```python
from build123d import *

# Parameters (mm, degrees)
EXTRUDE001_DEPTH               = 300
EXTRUDE002_DEPTH               = 300
EXTRUDE002_PLACEMENT_ANGLE     = 180
EXTRUDE004_DEPTH               = 2
EXTRUDE003_DEPTH               = 2
SKETCH_W                       = 449.952683
SKETCH_H                       = 299.978927
EXTRUDE_DEPTH                  = 2
FUSION_PLACEMENT_ANGLE         = 180
BASEFEATURE001_PLACEMENT_ANGLE = 180
POCKET001_DEPTH                = 825.012353
EXTRUDE005_DEPTH               = 450
POCKET_DEPTH                   = 250
POCKET002_DEPTH                = 500


with BuildPart() as right:
    # Wire → Extrude001 (new body)
    with BuildSketch(Plane(origin=(218.5150455, 150, 100.0712645), x_dir=(1, 0, 0), z_dir=(0, 1, 0))):
        Polygon((6.4963075, 100.0846805), (-3.4711005, 100.0846805), (-3.4711005, -98.1016935), (-6.4963075, -98.1016935), (-6.4963075, -98.7846775), (-5.4995125, -98.7846775), (-5.4995125, -99.4307345), (-6.4963075, -99.4307345), (-6.4963075, -100.0846805), (6.4963075, -100.0846805), (-1.4816445, -9.9001025), (-1.4816445, 10.1120285), (6.4963075, 98.0725005), align=None)
    extrude(amount=-EXTRUDE001_DEPTH)


with BuildPart() as left:
    # Wire001 → Extrude002 (new body)
    with BuildSketch(Plane(origin=(218.5150455, 150, 100.0712645), x_dir=(1, 0, 0), z_dir=(0, 1, 0))):
        Polygon((6.4963075, 100.0846805), (-3.4711005, 100.0846805), (-3.4711005, -98.1016935), (-6.4963075, -98.1016935), (-6.4963075, -98.7846775), (-5.4995125, -98.7846775), (-5.4995125, -99.4307345), (-6.4963075, -99.4307345), (-6.4963075, -100.0846805), (6.4963075, -100.0846805), (-1.4816445, -9.9001025), (-1.4816445, 10.1120285), (6.4963075, 98.0725005), align=None)
    extrude(amount=-EXTRUDE002_DEPTH)


with BuildPart() as left_1:
    # Extrude002 placement: moved
    add(left.part.rotate(Axis((0, 0, 0), (0, 0, 1)), EXTRUDE002_PLACEMENT_ANGLE))


with BuildPart() as inner_back_holder:
    # Sketch002 → Extrude004 (new body)
    with BuildSketch(Plane.XZ.offset(150)):
        Polygon((-213.019012, 3.99983), (-213.019012, 192.972672), (-216.785446, 192.972672), (-216.785446, 0.188954), (216.195801, 0.188954), (216.195801, 193.007004), (213.035522, 193.006973), (213.035522, 3.99983), align=None)
    extrude(amount=-EXTRUDE004_DEPTH)


with BuildPart() as inner_back_holder_1:
    # Extrude004 placement: moved
    add(inner_back_holder.part.moved(Location((0, 3, 0))))


with BuildPart() as outer_back_holder:
    # Sketch001 → Extrude003 (new body)
    with BuildSketch(Plane.XZ.offset(150)):
        Polygon((-213.019012, 3.99983), (-213.019012, 192.972672), (-216.785446, 192.972672), (-216.785446, 0.188954), (216.195801, 0.188954), (216.195801, 193.007004), (213.035522, 193.006973), (213.035522, 3.99983), align=None)
    extrude(amount=-EXTRUDE003_DEPTH)


with BuildPart() as main_body:
    # Sketch → Extrude (new body)
    with BuildSketch(Plane.XY):
        with Locations((-0.0037765, 0.0109025)):
            Rectangle(SKETCH_W, SKETCH_H)
    extrude(amount=EXTRUDE_DEPTH)

    # Fusion: union Right, Left, Inner-Back-Holder, Outer-Back-Holder
    add(right.part)
    add(left_1.part)
    add(inner_back_holder_1.part)
    add(outer_back_holder.part)


with BuildPart() as main_body_1:
    # Fusion placement: moved
    add(main_body.part.rotate(Axis((0, 0, 0), (0, 0, 1)), FUSION_PLACEMENT_ANGLE))


with BuildPart() as main_body_2:
    # BaseFeature001 placement: moved
    add(main_body_1.part.rotate(Axis((0, 0, 0), (0, 0, -1)), BASEFEATURE001_PLACEMENT_ANGLE))

    # Sketch004 → Pocket001 (cut, through all)
    with BuildSketch(Plane.YZ.offset(600)):
        Polygon((-150.000214, 200.026337), (-150.207199, 200.026337), (-150.207199, 2.124103), (-150, 2.124103), (-142.033401, 89.958923), (-142.033401, 109.971352), align=None)
    extrude(amount=-POCKET001_DEPTH, mode=Mode.SUBTRACT)


with BuildPart() as main_body001:
    # Wire002 → Extrude005 (new body)
    with BuildSketch(Plane(origin=(150, -218.5150455, 100.0712645), x_dir=(0, -1, 0), z_dir=(1, 0, 0))):
        Polygon((6.4963075, 100.0846805), (-3.4711005, 100.0846805), (-3.4711005, -98.1016935), (-6.4963075, -98.1016935), (-6.4963075, -98.7846775), (-5.4995125, -98.7846775), (-5.4995125, -99.4307345), (-6.4963075, -99.4307345), (-6.4963075, -100.0846805), (6.4963075, -100.0846805), (-1.4816445, -9.9001025), (-1.4816445, 10.1120285), (6.4963075, 98.0725005), align=None)
    extrude(amount=EXTRUDE005_DEPTH)


with BuildPart() as main_body001_1:
    # Extrude005 placement: moved
    add(main_body001.part.moved(Location((-375, 75, 0))))


with BuildPart() as main_body001_2:
    # BaseFeature placement: moved
    add(main_body001_1.part.moved(Location((375, -75, 0))))

    # Sketch003 → Pocket (cut, symmetric)
    with BuildSketch(Plane(origin=(375, 0, 0), x_dir=(1, 0, 0), z_dir=(0, -1, 0))):
        Polygon((-224.999924, 200.057419), (-217.03331, 109.971413), (-217.03331, 89.959267), (-224.999924, 2.122504), (-227.360413, 2.122504), (-227.360413, 200.057419), align=None)
    extrude(amount=POCKET_DEPTH, both=True, mode=Mode.SUBTRACT)

    # Sketch005 → Pocket002 (cut)
    with BuildSketch(Plane(origin=(375, -300, 0), x_dir=(1, 0, 0), z_dir=(0, -1, 0))):
        Polygon((225.000046, 200.027863), (225.188705, 200.027863), (225.188705, 2.123739), (225.000061, 2.123739), (217.034546, 89.959541), (217.034546, 109.969955), align=None)
    extrude(amount=-POCKET002_DEPTH, mode=Mode.SUBTRACT)


with BuildPart() as main_body001_3:
    # Body placement: moved
    add(main_body001_2.part.moved(Location((-375, 75, 0))))

    # Fusion001: union  Main Body
    add(main_body_2.part)


solid = main_body001_3.part
```
Geometry: final body of the model. Coordinates: model frame, mm. A direction names the side the tool comes from. Coordinates: 2 decimals unless noted, no trailing zeros. Answer in a Markdown table with one row per item. Add a question column.
Q1. Line query: L1, parallel to X at y = -72, z = 90; L2, parallel to Z at x = -163.5, y = 64; L3, parallel to X at y = 40, z = 15.5. Output: solid intervals per line, ascending.
Q2. Contact query for flat-ended pins moving along their axis: P1, Ø0.8, axis at x = -56, z = 198.5, coming from the +Y side; P2, Ø8, axis at x = 168, y = 16.5, coming from the +Z side; P3, Ø8, axis at x = 138, z = 154, coming from the -Y side. Output: stop coordinate, or through.
Q3. Mould query, pull axis Z, two halves, no side actions, for faces 1 (the flat face through (221.847, -143.6, 164.375)), 2 (the flat face through (216, 150, 99)), 3 (the flat face through (-3, 7, 0)). Classes: released by +Z, released by -Z, zero draft, split by the parting line, or undercut.
Q4. Reachability of faces 4 (the flat face through (-220.967, -2.1, 46.595)), 5 (the flat face through (-3, -142.033, 100)), 6 (the flat face through (215.044, 7, 99)), 7 (the flat face through (220.967, 2.1, 46.595)) from +Z, -Z, +X, -X, +Y, -Y: full face, straight path, thin tool, end or side. Return the list, or none.
Completed:
| question | item | result |
|---|---|---|
| 1 | L1 | x = -217.03 to -215.04, 215.04 to 217.03 |
| 1 | L2 | z = 0 to 2 |
| 1 | L3 | x = -223.79 to -215.04, 215.04 to 223.79 |
| 2 | P1 | stops at y = -137.02 |
| 2 | P2 | stops at z = 2 |
| 2 | P3 | stops at y = -146.28 |
| 3 | face 1 | undercut |
| 3 | face 2 | zero draft |
| 3 | face 3 | released by -Z |
| 4 | face 4 | -X, +Y, -Y |
| 4 | face 5 | +X, -X, -Y |
| 4 | face 6 | +Y |
| 4 | face 7 | +X, +Y, -Y |
